```python
from build123d import *

# Parameters (mm, degrees)
BOSS_EXTRUDE1_DEPTH = 225
FILLET1_R           = 2
FILLET2_R           = 2


with BuildPart() as part:
    # Sketch1 → Boss-Extrude1 (new body)
    with BuildSketch(Plane(origin=(0, 0, 0), x_dir=(0, 0, -1), z_dir=(1, 0, 0))):
        Polygon((-25.797072277, -87.459332388), (-25.797072277, -65.229332388), (413.812927723, -65.229332388), (413.812927723, -87.549332388), (412.812927723, -87.549332388), (412.812927723, -66.130301409), (-24.797072277, -66.130301409), (-24.797072277, -87.459332388), align=None)
    extrude(amount=BOSS_EXTRUDE1_DEPTH)

    # Fillet1
    fillet1_edges = [part.edges().sort_by_distance(p)[0] for p in [
        (112.5, -65.229332388, 25.797072277),
        (112.5, -65.229332388, -413.812927723),
    ]]
    fillet(fillet1_edges, radius=FILLET1_R)

    # Fillet2
    fillet2_edges = [part.edges().sort_by_distance(p)[0] for p in [
        (112.5, -66.130301409, -412.812927723),
        (112.5, -66.130301409, 24.797072277),
    ]]
    fillet(fillet2_edges, radius=FILLET2_R)


solid = part.part
```
Geometry check sheet. Reference: the model listing, model coordinates, mm. A direction names the side the tool comes from. Coordinates: 2 decimals unless noted, no trailing zeros. Write each loop counter-clockwise with the first axis right and the second up, starting at its lowest first coordinate (ties: lowest second). Pieces come first, ordered by that corner, then holes. Notation, with made-up numbers: M -4,-9.75 L 34,-9.75 A28 cw 34,24.25 Z; hole C 74,-10.75 d4. An arc over 180 degrees is marked long. Use one line per item in the form item = value. Start each with the question number.
1) Thickness scan on probe 1 along Z at (x, y) = (173, -72.5); probe 2 along Y at (x, z) = (144, -171.5); probe 3 along Z at (x, y) = (141, -66.75). Record the ranges inside material, lowest first. Write a range as from..to.
2) Section check A-A on y = -76.5. Enter the section's corners in (x, z), and give its area (3 significant figures).
3) Set-up check for faces 1 (the flat face through (0, -65.6, -195)), 2 (the flat face through (111, -66.13, -197)): record each of +Z, -Z, +X, -X, +Y, -Y from which the full face is reachable in a straight line by a thin tool's end or side.
4) Section check C-C on z = -115. Enter the section's corners in (x, y), and give its area (3 significant figures).
5) Release check for a two-part mould opening along Z. For faces 3 (the flat face through (111, -78, -412.813)), 4 (the flat face through (111, -65.229, -191)), 5 (the flat face through (111, -77, -413.813)) record: pulls with the +Z half, pulls with the -Z half, needs draft (parallel to the pull), parting line crosses it, or undercut.
6) Go/stop test with flat-tipped pins: pin 1 Ø8 at (x, z) = (87, -220.5) entering from -Y; pin 2 Ø1.1 at (x, z) = (122.5, 25) entering from -Y. Record where each tip stops, or that it passes through.
7) Section check B-B on x = 55. Enter the section's corners in (y, z).
Responses:
q1.probe_1 = -413.81..-412.81, 24.8..25.8
q1.probe_2 = -66.13..-65.23
q1.probe_3 = -413.75..-412.26, 24.24..25.74
q2.outline = M 0,-413.81 L 225,-413.81 L 225,-412.81 L 0,-412.81 Z; M 0,24.8 L 225,24.8 L 225,25.8 L 0,25.8 Z
q2.area = 450 mm2
q3.face_1 = +Z, -Z, -X, +Y, -Y
q3.face_2 = +X, -X, -Y
q4.outline = M 0,-66.13 L 225,-66.13 L 225,-65.23 L 0,-65.23 Z
q4.area = 203 mm2
q5.face_3 = undercut
q5.face_4 = needs draft
q5.face_5 = pulls with the -Z half
q6.pin_1 = -66.13
q6.pin_2 = -87.46
q7.outline = M -87.55,-413.81 L -67.23,-413.81 A2 ccw -65.23,-411.81 L -65.23,23.8 A2 ccw -67.23,25.8 L -87.46,25.8 L -87.46,24.8 L -68.13,24.8 A2 cw -66.13,22.8 L -66.13,-410.81 A2 cw -68.13,-412.81 L -87.55,-412.81 Z
